from build123d import *

# Parameters (mm, degrees)
EXTRUDE_1_DEPTH             = 10
EXTRUDE_2_DEPTH             = 12
FILLET_1_R                  = 6
FILLET_2_R                  = 1.49
HOLE_WIZARD_M44_D           = 4.3
HOLE_WIZARD_M44_CSINK_D     = 8.7
HOLE_WIZARD_M44_CSINK_ANGLE = 90
HOLE_WIZARD_4_0_2_D         = 4
HOLE_WIZARD_4_0_2_DEPTH     = 6
HOLE_WIZARD_4_0_2_TIP       = 1.2017212380551205
HOLE_WIZARD_7_0_7_1_D       = 7
HOLE_WIZARD_7_0_7_1_DEPTH   = 6
HOLE_WIZARD_7_0_7_1_TIP     = 2.103012166596461
SKETCH_54_R                 = 6.999999999999999
CUT_EXTRUDE_5_DEPTH         = 2
HOLE_WIZARD_M2_21_D         = 2
HOLE_WIZARD_M2_21_DEPTH     = 10
HOLE_WIZARD_M2_21_TIP       = 0.6008606190275603
CUT_EXTRUDE_11_DEPTH        = 4
HOLE_WIZARD_M2_22_D         = 2
HOLE_WIZARD_M2_22_DEPTH     = 10
HOLE_WIZARD_M2_22_TIP       = 0.6008606190275603
CUT_EXTRUDE_12_DEPTH        = 4


with BuildPart() as part:
    # Эскиз1 → Бобышка-Вытянуть1 (new body)
    with BuildSketch(Plane.XY):
        Polygon((0, 0), (64, 0), (64.00000000000001, 34.01923788646688), (48.99999999999994, 59.99999999999999), (14.999999999999943, 59.99999999999999), (0, 34.02), align=None)
    extrude(amount=EXTRUDE_1_DEPTH)

    # Эскиз3 → Бобышка-Вытянуть2 (add)
    with BuildSketch(Plane.XY.offset(10)):
        Polygon((0, 0), (64, 0), (64.00000000000001, 34.01923788646688), (58.29037785163881, 43.90859353944907), (57, 43.16359353944907), (60.99999999999999, 36.23539030917355), (61.00000000000001, 9.999999999999998), (6.000000000000005, 9.999999999999993), (6, 41.43206556072121), (8.000044001452048, 44.896141771236174), (6.709675613035229, 45.64115816177706), (0, 34.02), align=None)
    extrude(amount=EXTRUDE_2_DEPTH)

    # Скругление1
    fillet_1_edges = [part.edges().sort_by_distance(p)[0] for p in [
        (0, 34.02, 11),
        (14.999999999999943, 59.99999999999999, 5),
        (48.99999999999994, 59.99999999999999, 5),
        (64.00000000000001, 34.01923788646688, 11),
        (64, 0, 11),
        (0, 0, 11),
    ]]
    fillet(fillet_1_edges, radius=FILLET_1_R)

    # Скругление2
    fillet_2_edges = [part.edges().sort_by_distance(p)[0] for p in [
        (58.29037785163881, 43.90859353944907, 16),
        (6.709675613035229, 45.64115816177706, 16),
    ]]
    fillet(fillet_2_edges, radius=FILLET_2_R - 0.0001)  # a hair under: the kernel refuses the full size

    # Зенковка для  винта с плоской головкой M44 (through all)
    with Locations(Plane(origin=(0, 0, 0), x_dir=(-1, 0, 0), z_dir=(0, 0, -1))):
        with Locations((-5.999949191, 6), (-58, 6), (-31.999974596, 49)):
            CounterSinkHole(HOLE_WIZARD_M44_D / 2, HOLE_WIZARD_M44_CSINK_D / 2, counter_sink_angle=HOLE_WIZARD_M44_CSINK_ANGLE)

    # Отверстия под штифты Ø4.0 мм2
    with Locations(Plane(origin=(0, 0, 10), x_dir=(-1, 0, 0), z_dir=(0, 0, 1))):
        with Locations((-36.5, -55), (-27.499949191, -55)):
            Hole(HOLE_WIZARD_4_0_2_D / 2, depth=HOLE_WIZARD_4_0_2_DEPTH)
            with Locations((0, 0, -(HOLE_WIZARD_4_0_2_DEPTH + HOLE_WIZARD_4_0_2_TIP / 2))):  # 118° drill point
                Cone(0, HOLE_WIZARD_4_0_2_D / 2, HOLE_WIZARD_4_0_2_TIP, mode=Mode.SUBTRACT)

    # Диаметр отверстия Ø7.0 (7)1
    with Locations(Plane(origin=(0, 0, 10), x_dir=(-1, 0, 0), z_dir=(0, 0, 1))):
        with Locations((-44.05, -39), (-19.949949191, -39)):
            Hole(HOLE_WIZARD_7_0_7_1_D / 2, depth=HOLE_WIZARD_7_0_7_1_DEPTH)
            with Locations((0, 0, -(HOLE_WIZARD_7_0_7_1_DEPTH + HOLE_WIZARD_7_0_7_1_TIP / 2))):  # 118° drill point
                Cone(0, HOLE_WIZARD_7_0_7_1_D / 2, HOLE_WIZARD_7_0_7_1_TIP, mode=Mode.SUBTRACT)

    # Эскиз54 → Вырез-Вытянуть5 (cut)
    with BuildSketch(Plane.XY.offset(10)):
        with Locations((44.050000000000004, 21)):
            Circle(SKETCH_54_R)
    extrude(amount=-CUT_EXTRUDE_5_DEPTH, mode=Mode.SUBTRACT)

    # Сверло под метчик  спиральное M2.21
    with Locations(Plane(origin=(0, 0, 0), x_dir=(-1, 0, 0), z_dir=(0, -1, 0))):
        with Locations((-26, -18), (-38, -18)):
            Hole(HOLE_WIZARD_M2_21_D / 2, depth=HOLE_WIZARD_M2_21_DEPTH)
            with Locations((0, 0, -(HOLE_WIZARD_M2_21_DEPTH + HOLE_WIZARD_M2_21_TIP / 2))):  # 118° drill point
                Cone(0, HOLE_WIZARD_M2_21_D / 2, HOLE_WIZARD_M2_21_TIP, mode=Mode.SUBTRACT)

    # Эскиз58 → Вырез-Вытянуть11 (cut)
    with BuildSketch(Plane(origin=(-9.5e-16, 9.999999999999993, 0), x_dir=(1, 9e-17, 0), z_dir=(-9e-17, 1, 0))):
        Polygon((28.309401076758505, -17.999999999999993), (27.154700538379252, -15.99999999999999), (24.845299461620748, -15.999999999999986), (23.690598923241495, -17.999999999999986), (24.845299461620744, -19.999999999999982), (27.154700538379256, -19.999999999999986), align=None)
        Polygon((40.3094010767585, -17.999999999999993), (39.154700538379245, -15.999999999999993), (36.845299461620755, -15.99999999999999), (35.6905989232415, -17.999999999999996), (36.84529946162075, -19.999999999999993), (39.15470053837924, -19.999999999999996), align=None)
    extrude(amount=-CUT_EXTRUDE_11_DEPTH, mode=Mode.SUBTRACT)

    # Сверло под метчик  спиральное M2.22
    with Locations(Plane(origin=(0, 0, 0), x_dir=(-1, 0, 0), z_dir=(0, -1, 0))):
        with Locations((-32, -12)):
            Hole(HOLE_WIZARD_M2_22_D / 2, depth=HOLE_WIZARD_M2_22_DEPTH)
            with Locations((0, 0, -(HOLE_WIZARD_M2_22_DEPTH + HOLE_WIZARD_M2_22_TIP / 2))):  # 118° drill point
                Cone(0, HOLE_WIZARD_M2_22_D / 2, HOLE_WIZARD_M2_22_TIP, mode=Mode.SUBTRACT)

    # Эскиз61 → Вырез-Вытянуть12 (cut)
    with BuildSketch(Plane(origin=(-9.5e-16, 9.999999999999993, 0), x_dir=(1, 9e-17, 0), z_dir=(-9e-17, 1, 0))):
        Polygon((34.3094010767585, -11.999999999999998), (33.15470053837925, -10.000000000000002), (30.84529946162075, -9.999999999999998), (29.690598923241495, -11.999999999999996), (30.845299461620744, -13.999999999999996), (33.15470053837924, -14), align=None)
    extrude(amount=-CUT_EXTRUDE_12_DEPTH, mode=Mode.SUBTRACT)


solid = part.part
Work out the finished part from the listing and answer in its coordinate system (mm). A direction names the side the tool comes from. Round coordinates to 2 decimals unless told otherwise and drop trailing zeros. Write each loop counter-clockwise with the first axis right and the second up, starting at its lowest first coordinate (ties: lowest second). Pieces come first, ordered by that corner, then holes. Notation, with made-up numbers: M -9,20 L 47,20 A15 cw 47,40 Z; hole C 18,-32 d9. An arc over 180 degrees is marked long. Use a Markdown table: item, result.
1) Which of the six approach directions +Z, -Z, +X, -X, +Y, -Y give full straight-line access (tool end or side, diameter ignored) to faces 5 (the face through (61, 23, 16)), 6 (the face through (30.415, 50.453, 6.155)), 7 (the face through (30.276, 8.028, 10.986))?
Taken from the geometry:
| item | result |
|---|---|
| face 5 | +Z |
| face 6 | +Z, -Z |
| face 7 | +Y |
2) Determine the mould class of faces 1 (the face through (38, 3, 19)), 2 (the face through (31.6, 0, 10.8)), 3 (the face through (58.436, 43.656, 8.402)), 4 (the face through (38, 8, 16)) for opening direction X: pulls with the +X half, pulls with the -X half, needs draft (parallel to the pull), parting line crosses it, or undercut.
Taken from the geometry:
| item | result |
|---|---|
| face 1 | undercut |
| face 2 | needs draft |
| face 3 | pulls with the +X half |
| face 4 | undercut |
3) The part is cut by section B-B on y = 13. Give the vertices of the cut face in (x, z).
Taken from the geometry:
| item | result |
|---|---|
| outline | M 0,0 L 64,0 L 64,22 L 61,22 L 61,10 L 6,10 L 6,22 L 0,22 Z |
4) The part is cut by section A-A on z = 20.75. State how many separate pieces and enclosed holes the cut face has, plus the area to 3 significant figures.
Taken from the geometry:
| item | result |
|---|---|
| separate pieces | 1 |
| enclosed holes | 2 |
| area | 863 mm2 |
5) Consider line 1 (X direction, y = 6, z = 3.75); line 2 (Y direction, x = 44.05, z = 8.95); line 3 (Z direction, x = 38, y = 3.55). Determine where each line is inside the solid, lowest interval first. Write a range as [from, to].
Taken from the geometry:
| item | result |
|---|---|
| line 1 | x = [0, 3.85], [8.15, 55.85], [60.15, 64] |
| line 2 | y = [0, 14], [28, 35.5], [42.5, 60] |
| line 3 | z = [0, 17], [19, 22] |
6) The part is cut by section D-D on y = 49. Give the vertices of the cut face in (x, z).
Taken from the geometry:
| item | result |
|---|---|
| outline | M 8.65,0 L 27.65,0 L 29.85,2.2 L 29.85,10 L 8.65,10 Z; M 34.15,2.2 L 36.35,0 L 55.35,0 L 55.35,10 L 34.15,10 Z |
7) Flat-ended cylindrical pins translate along their axes: pin 1 (4 mm diameter, centred on x = 19.95, y = 39, fed in from +Z); pin 2 (3.5 mm diameter, centred on x = 21.5, z = 16, fed in from +Y); pin 3 (2 mm diameter, centred on x = 52, y = 45, fed in from +Z). Find the tip coordinate at first contact, or state that the pin passes through.
Taken from the geometry:
| item | result |
|---|---|
| pin 1 | stops at z = 3.1 |
| pin 2 | stops at y = 10 |
| pin 3 | stops at z = 10 |
